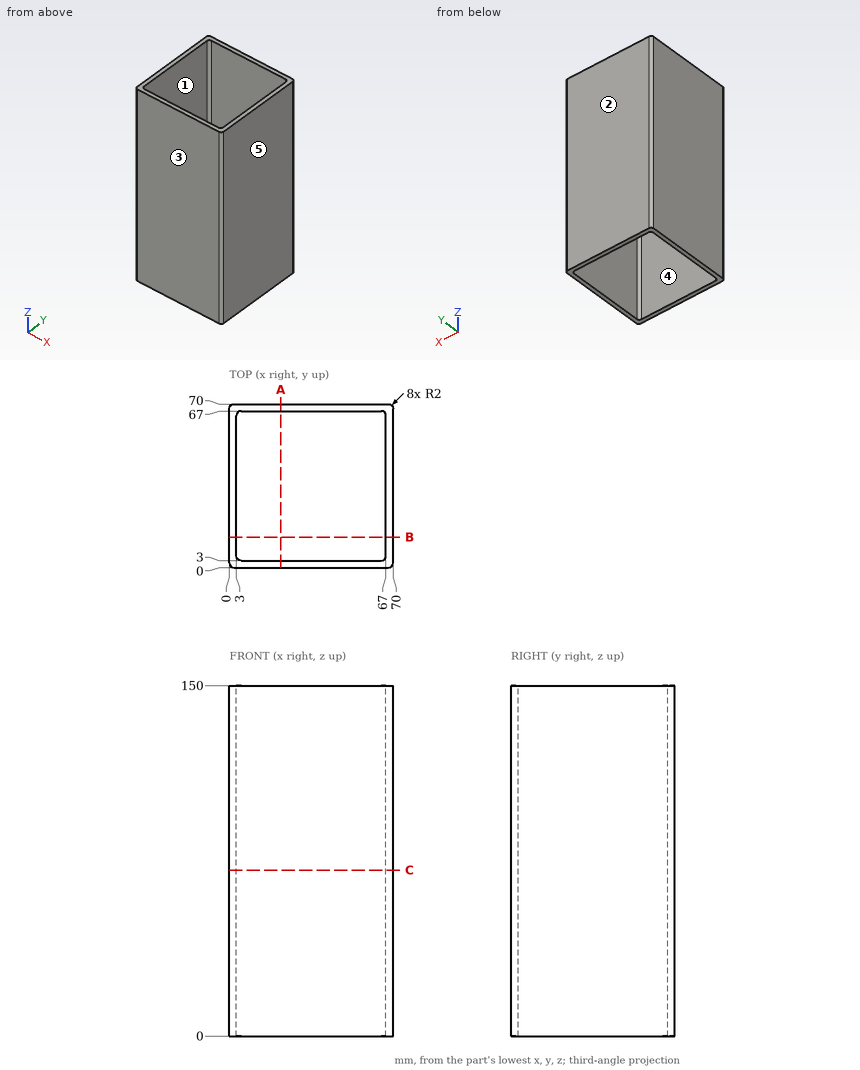
Here's the drawing with two shaded views (mm, measured from the low corner). I have some questions. A direction names the side the tool comes from. Round coordinates to 2 decimals unless told otherwise and drop trailing zeros. Write each loop counter-clockwise with the first axis right and the second up, starting at its lowest first coordinate (ties: lowest second). Pieces come first, ordered by that corner, then holes.
(1) If I drill on probe 1 along Y at (x, z) = (18, 25); probe 2 along Y at (x, z) = (3.5, 56.5), over which ranges is the centre line in solid material (lowest first)?
Findings below:
probe 1: y = 0 to 3, 67 to 70
probe 2: y = 0 to 3.68, 66.32 to 70
(2) Suppose I cut it at A-A on x = 22. Write out the boundary of the cut face in (y, z).
Findings below:
outline: (0, 0) - (3, 0) - (3, 150) - (0, 150) - close; (67, 0) - (70, 0) - (70, 150) - (67, 150) - close
(3) Suppose I cut it at C-C on z = 71. Write out the boundary of the cut face in (x, y), and give its area (3 significant figures).
Findings below:
outline: (0, 2) arc R2 ccw to (2, 0) - (68, 0) arc R2 ccw to (70, 2) - (70, 68) arc R2 ccw to (68, 70) - (2, 70) arc R2 ccw to (0, 68) - close; hole (3, 5) arc R2 ccw to (5, 3) - (65, 3) arc R2 ccw to (67, 5) - (67, 65) arc R2 ccw to (65, 67) - (5, 67) arc R2 ccw to (3, 65) - close
area: 804 mm2
(4) Thinking about a two-plate mould opening in Y: for the marked faces 3, 4 and 5, which applies, +Y half, -Y half, draft (parallel to the pull), parting line (faces both ways), or undercut?
Findings below:
face 3: -Y half
face 4: undercut
face 5: draft
(5) Which directions (+Z, -Z, +X, -X, +Y, -Y) give clear straight access to the entire face, cutting with the end or side of a thin tool? Please do the marked faces 1 and 2.
Findings below:
face 1: +Z, -Z
face 2: +Z, -Z, +X, -X, +Y
